The model under review builds one solid part; all positions refer to its coordinate system, in mm. Face numbers are marked on the shaded views. Round coordinates to 2 decimals unless told otherwise and drop trailing zeros. Order: outer loops, then holes, each group sorted by start corner. A loop starts at its lowest first (then second) coordinate and runs counter-clockwise, first axis right, second up.
1) Consider section A-A (z = 40). Give the boundary of the cut face in (x, y) (3 decimals).
2) To check wall thickness, follow L1, parallel to Y at x = 0, z = 30 (3 decimals); L2, parallel to Z at x = 0.5, y = 3.5; L3, parallel to X at y = 3, z = 38.5. State the ranges of each line that lie inside material, in increasing order.
3) Mouldability with a two-part tool opening along X and no side actions: class the marked faces 1, 2 and 3 as pulls with the +X half, pulls with the -X half, needs draft (parallel to the pull), parting line crosses it, or undercut.
4) Clearance check with flat-ended pins moving along their axes: P1, Ø6, axis at y = -6, z = 39, coming from the +X side; P2, Ø5, axis at x = 0.5, y = 0.5, coming from the +Z side; P3, Ø5, axis at x = 7, z = 21.5, coming from the +Y side (3 decimals). State where each tip first meets the part, or that it passes through.
from build123d import *

# Parameters (mm, degrees)
F0_R     = 3.175
F1_DEPTH = 12.7
F2_R     = 9.525
F3_DEPTH = 38.1
F4_R     = 5.08
F5_R     = 6.35
F6_DEPTH = 31.75


with BuildPart() as f1:
    # F0 (on Top) → F1 (new body)
    with BuildSketch(Plane.XY):
        Circle(F0_R)
    extrude(amount=F1_DEPTH)

    # F2 (on face) → F3 (join)
    with BuildSketch(Plane.XY.offset(12.7)):
        Circle(F2_R)
    extrude(amount=F3_DEPTH)

    # F4
    f4_edges = [f1.edges().sort_by_distance(p)[0] for p in [
        (-9.525, 0, 50.8),
        (-9.525, 0, 12.7),
    ]]
    fillet(f4_edges, radius=F4_R)

    # F5 (on face) → F6 (cut)
    with BuildSketch(Plane.XY.offset(50.8)):
        Circle(F5_R)
    extrude(amount=-F6_DEPTH, mode=Mode.SUBTRACT)


solid = f1.part
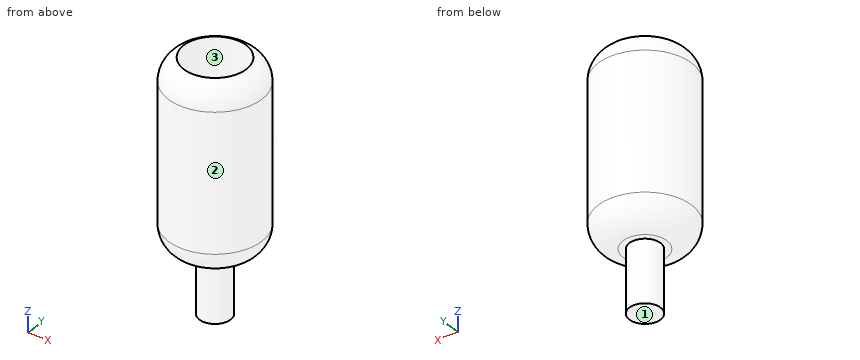
Answer below:
1. outline: circle Ø19.05 at (0, 0); hole circle Ø12.7 at (0, 0)
2. L1: y = -9.525 to -6.35, 6.35 to 9.525
2. L2: z = 12.7 to 19.05
2. L3: x = -9.04 to -5.6, 5.6 to 9.04
3. face 1: needs draft
3. face 2: parting line crosses it
3. face 3: undercut
4. P1: stops at x = 9.04
4. P2: stops at z = 19.05
4. P3: stops at y = 8.395
